Source: CAD feature listing. Evaluate the final solid. Frame: model axes, mm. Face numbers are marked on the shaded views. Give positions to 0.01 mm unless a question says otherwise; leave off trailing zeros. Loops run counter-clockwise (first coordinate to the right, second up) from the corner with the lowest first, then second, coordinate; pieces in that order, holes last. Notation, with made-up numbers: M 42.25,2.25 L 53.25,2.25 A16 cw 53.25,28.25 Z; hole C 10.25,-30 d3. An arc over 180 degrees is marked long. Answer in a Markdown table with one row per item.
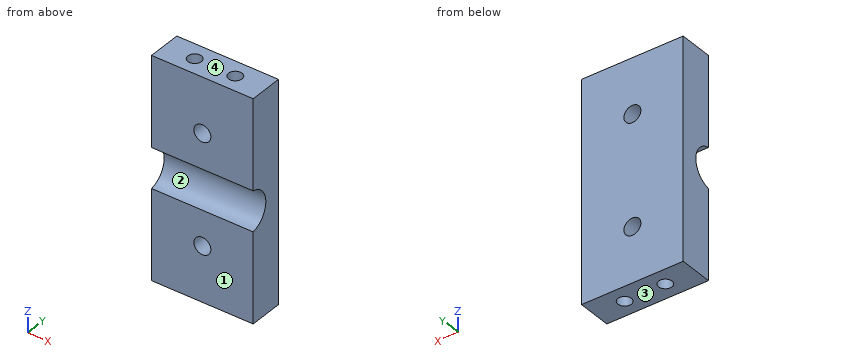
```python
from build123d import *

# Parameters (mm, degrees)
SKETCH_1_W            = 30
SKETCH_1_H            = 65
EXTRUDE_1_DEPTH       = 10
SKETCH_2_R            = 6
CUT_EXTRUDE_2_DEPTH   = 73.284161474
SKETCH_3_R            = 2.5
CUT_EXTRUDE_3_DEPTH   = 73.284161474
SKETCH_4_R            = 2
CUT_EXTRUDE_1_DEPTH   = 20
CUT_EXTRUDE_START     = -20
SKETCH_5_R            = 2
CUT_EXTRUDE_2_2_DEPTH = 20


with BuildPart() as part:
    # Эскиз1 → Вытянуть1 (new body)
    with BuildSketch(Plane(origin=(0, 0, 0), x_dir=(1, 0, 0), z_dir=(0, 1, 0))):
        with Locations((15, 32.5)):
            Rectangle(SKETCH_1_W, SKETCH_1_H)
    extrude(amount=EXTRUDE_1_DEPTH)

    # Эскиз2 → Cut-Extrude 2 (cut, through all)
    with BuildSketch(Plane(origin=(30, 0, 0), x_dir=(0, 0, -1), z_dir=(1, 0, 0))):
        with Locations((32.5, -1)):
            Circle(SKETCH_2_R)
    extrude(amount=-CUT_EXTRUDE_2_DEPTH, mode=Mode.SUBTRACT)

    # Эскиз3 → Вытянуть3 (cut, through all)
    with BuildSketch(Plane(origin=(0, 10, 0), x_dir=(1, 0, 0), z_dir=(0, 1, 0))):
        with Locations(Location((15, 48.75, 0), (0, 0, 270))):
            Circle(SKETCH_3_R)
        with Locations(Location((15, 16.25, 0), (0, 0, 270))):
            Circle(SKETCH_3_R)
    extrude(amount=-CUT_EXTRUDE_3_DEPTH, mode=Mode.SUBTRACT)

    # Эскиз4 → Вырез-Вытянуть1 (cut)
    with BuildSketch(Plane.XY):
        with Locations((9, 5.000000757)):
            Circle(SKETCH_4_R)
        with Locations((21, 5.000000757)):
            Circle(SKETCH_4_R)
    extrude(amount=-CUT_EXTRUDE_1_DEPTH, mode=Mode.SUBTRACT)

    # Эскиз5 → Cut-Extrude 2 2 (cut)
    with BuildSketch(Plane(origin=(0, 0, -65), x_dir=(-1, 0, 0), z_dir=(0, 0, -1)).offset(CUT_EXTRUDE_START)):
        with Locations(Location((-20.999999999, 5.000000369, 0), (0, 0, 179.99998886))):
            Circle(SKETCH_5_R)
        with Locations(Location((-8.999999999, 5.000000369, 0), (0, 0, 179.99998886))):
            Circle(SKETCH_5_R)
    extrude(amount=CUT_EXTRUDE_2_2_DEPTH, mode=Mode.SUBTRACT)


solid = part.part
```
1) Section B-B, the plane x = 21. Return loops of the section in (y, z).
Reply:
| item | result |
|---|---|
| outline | M 0,-65 L 3,-65 L 3,-45 L 7,-45 L 7,-65 L 10,-65 L 10,0 L 7,0 L 7,-20 L 3,-20 L 3,0 L 0,0 L 0,-26.58 A6 cw 0,-38.42 Z |
2) Pull-direction query (Z, two-part tool) for the marked faces 1, 2, 3 and 4; classes: released by +Z, released by -Z, zero draft, split by the parting line, or undercut.
Reply:
| item | result |
|---|---|
| face 1 | zero draft |
| face 2 | undercut |
| face 3 | released by -Z |
| face 4 | released by +Z |
3) Section C-C, the plane z = -6.5. Return loops of the section in (x, y).
Reply:
| item | result |
|---|---|
| outline | M 0,0 L 30,0 L 30,10 L 0,10 Z; hole C 9,5 d4; hole C 21,5 d4 |
4) Section A-A, the plane z = -48.75. Return loops of the section in (x, y).
Reply:
| item | result |
|---|---|
| outline | M 0,0 L 12.5,0 L 12.5,10 L 0,10 Z; M 17.5,0 L 30,0 L 30,10 L 17.5,10 Z; hole C 9,5 d4; hole C 21,5 d4 |
5) Section D-D, the plane x = 14. Return loops of the section in (y, z), then the cut area to 3 significant figures.
Reply:
| item | result |
|---|---|
| outline | M 0,-65 L 10,-65 L 10,-51.04 L 0,-51.04 Z; M 0,-46.46 L 10,-46.46 L 10,-18.54 L 0,-18.54 L 0,-26.58 A6 cw 0,-38.42 Z; M 0,-13.96 L 10,-13.96 L 10,0 L 0,0 Z |
| area | 514 mm² |
6) Material intervals for L1, parallel to X at y = 6, z = -48.75; L2, parallel to Y at x = 9, z = -56.5; L3, parallel to Z at x = 14.5, y = 1, sorted ascending.
Reply:
| item | result |
|---|---|
| L1 | x = 0 to 7.27, 10.73 to 12.5, 17.5 to 19.27, 22.73 to 30 |
| L2 | y = 0 to 3, 7 to 10 |
| L3 | z = -65 to -51.2, -46.3 to -38.16, -26.84 to -18.7, -13.8 to 0 |
7) Pin query (flat end, axial travel): pin 1 Ø3 at (x, z) = (15, -48.75) entering from +Y; pin 2 Ø2.5 at (x, y) = (9, 5) entering from -Z; pin 3 Ø1.2 at (x, y) = (20, 5.5) entering from +Z. Return the tip coordinate at first contact, or that it passes through.
Reply:
| item | result |
|---|---|
| pin 1 | passes through |
| pin 2 | stops at z = -45 |
| pin 3 | stops at z = -20 |
